from build123d import *

# Parameters (mm, degrees)
SKETCH1_R           = 28.4
BOSS_EXTRUDE1_DEPTH = 3
SKETCH2_R           = 11
BOSS_EXTRUDE2_DEPTH = 20
SKETCH3_R           = 5
CUT_EXTRUDE1_DEPTH  = 24
SKETCH4_R           = 2
CUT_EXTRUDE2_DEPTH  = 15
CHAMFER1_SIZE       = 1
SKETCH5_R           = 2
CUT_EXTRUDE5_DEPTH  = 4.0000001
CIRPATTERN2_COUNT   = 12


with BuildPart() as part:
    # Sketch1 → Boss-Extrude1 (new body)
    with BuildSketch(Plane.XY):
        Circle(SKETCH1_R)
    extrude(amount=BOSS_EXTRUDE1_DEPTH)

    # Sketch2 → Boss-Extrude2 (add)
    with BuildSketch(Plane.XY.offset(3)):
        Circle(SKETCH2_R)
    extrude(amount=BOSS_EXTRUDE2_DEPTH)

    # Sketch3 → Cut-Extrude1 (cut, through all)
    with BuildSketch(Plane.XY.offset(23)):
        Circle(SKETCH3_R)
    extrude(amount=-CUT_EXTRUDE1_DEPTH, mode=Mode.SUBTRACT)

    # Sketch4 → Cut-Extrude2 (cut)
    with BuildSketch(Plane(origin=(0, 0, 0), x_dir=(1, 0, 0), z_dir=(0, 1, 0))):
        with Locations((0, -15)):
            Circle(SKETCH4_R)
    extrude(amount=-CUT_EXTRUDE2_DEPTH, mode=Mode.SUBTRACT)

    # Chamfer1
    chamfer1_edges = [part.edges().sort_by_distance(p)[0] for p in [
        (-11, 0, 3),
        (-11, 0, 23),
    ]]
    chamfer(chamfer1_edges, length=CHAMFER1_SIZE)

    # Sketch5 → Cut-Extrude5 (cut, through all)
    with BuildSketch(Plane.XY.offset(3)):
        with Locations((11.9, 20.61140461)):
            Circle(SKETCH5_R)
    cut_extrude5 = extrude(amount=-CUT_EXTRUDE5_DEPTH, mode=Mode.SUBTRACT)

    # CirPattern2: Cut-Extrude5 ×12 about axis
    cirpattern2_axis = Axis((0, 0, 0), (0, 0, 1))
    for i in range(1, CIRPATTERN2_COUNT):
        add(cut_extrude5.rotate(cirpattern2_axis, i * 360 / CIRPATTERN2_COUNT), mode=Mode.SUBTRACT)


solid = part.part
Here's how the part is built. I have some questions about the finished solid (model axes, mm). A direction names the side the tool comes from. Give positions to 0.01 mm unless a question says otherwise; leave off trailing zeros. Loops run counter-clockwise (first coordinate to the right, second up) from the corner with the lowest first, then second, coordinate; pieces in that order, holes last. Notation, with made-up numbers: (-40, -30) -> (-9, -30) arc R26 cw to (-9, 0) -> close; hole circle Ø9 at (55.25, -19.5). An arc over 180 degrees is marked (long way). Answer as a JSON object with one key per item and string values. Group by question number.
Item 1: Imagine slicing it at A-A on x = 0. Write out the boundary of the cut face in (y, z).
Item 2: On a 3-axis mill with a long thin cutter (end or side, diameter ignored), from which of +Z, -Z, +X, -X, +Y, -Y can I reach the whole of each face in a straight line? I mean faces 5 (the cylindrical face through (-2.38, -10.74, 12.87)), 6 (the cylindrical face through (0, -8, 13)), 7 (the cylindrical face through (-12.975, 18.925, 1.521)). Say none if no direction works.
Item 3: Will these pins go through, and if not, where does the flat tip stop? pin 1 (2.5 mm diameter, centred on x = -20.61, y = -11.9, fed in from +Z); pin 2 (6.5 mm diameter, centred on x = 0, z = 15, fed in from -Y); pin 3 (12 mm diameter, centred on y = -3, z = 14, fed in from -X); pin 4 (8 mm diameter, centred on x = -5.5, z = 19, fed in from +Y).
Item 4: Thinking about a two-plate mould opening in X: for faces 1 (the cylindrical face through (-3.697, 28.158, 1.479)), 2 (the flat face through (2, 5, 23)), 3 (the cylindrical face through (25.798, -0.088, 1.521)), 4 (the cylindrical face through (10.426, -19.26, 1.521)), which applies, pulls with the +X half, pulls with the -X half, needs draft (parallel to the pull), parting line crosses it, or undercut?
Item 5: Imagine slicing it at B-B on y = 23.8. Write out the boundary of the cut face in (x, z), then the cut area to 3 significant figures.
Item 6: I need wall thicknesses on L1, parallel to Y at x = 11.9, z = 0.7; L2, parallel to Z at x = 21.5, y = -18. Which ranges of each line are inside material? Lowest first, please.
Item 7: Imagine slicing it at D-D on z = 5.25. Write out the boundary of the cut face in (x, y), then the cut area to 3 significant figures.
Answer list:
{
 "1": {"outline": "(-28.4, 0) -> (-25.8, 0) -> (-25.8, 3) -> (-28.4, 3) -> close; (-21.8, 0) -> (-5, 0) -> (-5, 13) -> (-11, 13) -> (-11, 4) -> (-12, 3) -> (-21.8, 3) -> close; (-11, 17) -> (-5, 17) -> (-5, 23) -> (-10, 23) -> (-11, 22) -> close; (5, 0) -> (21.8, 0) -> (21.8, 3) -> (12, 3) -> (11, 4) -> (11, 22) -> (10, 23) -> (5, 23) -> close; (25.8, 0) -> (28.4, 0) -> (28.4, 3) -> (25.8, 3) -> close"},
 "2": {"face 5": "+Z", "face 6": "-Y", "face 7": "+Z, -Z"},
 "3": {"pin 1": "passes through", "pin 2": "stops at y = -11", "pin 3": "stops at x = -11", "pin 4": "stops at y = 10.9"},
 "4": {"face 1": "parting line crosses it", "face 2": "needs draft", "face 3": "undercut", "face 4": "undercut"},
 "5": {"outline": "(-15.5, 0) -> (-2, 0) -> (-2, 3) -> (-15.5, 3) -> close; (2, 0) -> (15.5, 0) -> (15.5, 3) -> (2, 3) -> close", "area": "81.0 mm2"},
 "6": {"L1": "y = -25.79 to -22.61, -18.61 to 18.61, 22.61 to 25.79", "L2": "z = 0 to 3"},
 "7": {"outline": "circle Ø22 at (0, 0); hole circle Ø10 at (0, 0)", "area": "302 mm2"}
}
